Geometry: final body of the model. Coordinates: model frame, mm. Round coordinates to 2 decimals unless told otherwise and drop trailing zeros. Loops run counter-clockwise (first coordinate to the right, second up) from the corner with the lowest first, then second, coordinate; pieces in that order, holes last. Notation, with made-up numbers: M -16,33 L 16,33 A21 ccw 16,48 Z; hole C -20,76.25 d7. An arc over 180 degrees is marked long. Return JSON: item names as keys, results as strings.
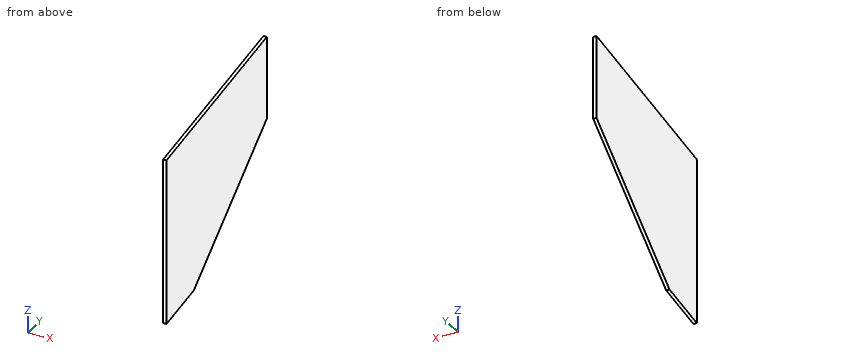
from build123d import *

# Parameters (mm, degrees)
BOSS_EXTRUDE1_DEPTH      = 1.27
BOSS_EXTRUDE1_DEPTH_BACK = 1.27


with BuildPart() as part:
    # Sketch1 → Boss-Extrude1 (new body, two sides)
    with BuildSketch(Plane(origin=(0, 0, 0), x_dir=(0, 0, -1), z_dir=(1, 0, 0))) as boss_extrude1_sk:
        Polygon((0, 0), (127, 0), (120.281942035, 38.1), (38.867120795, 139.7), (-24.632879205, 139.7), align=None)
    extrude(amount=BOSS_EXTRUDE1_DEPTH)
    extrude(boss_extrude1_sk.sketch, amount=-BOSS_EXTRUDE1_DEPTH_BACK)


solid = part.part
Q1. Section query A-A (x = -0.2). Output: boundary loops of the cut face in (y, z).
Determined:
{"outline": "M 0,-127 L 38.1,-120.28 L 139.7,-38.87 L 139.7,24.63 L 0,0 Z"}
Q2. Section query B-B (y = 46.5). Output: boundary loops of the cut face in (x, z), plus the area to 3 significant figures.
Determined:
{"outline": "M -1.27,-113.55 L 1.27,-113.55 L 1.27,8.2 L -1.27,8.2 Z", "area": "309 mm^2"}
Q3. Pin query (flat end, axial travel): pin 1 (1.5 mm diameter, centred on x = 0, y = 84, fed in from -Z). Return the tip coordinate at first contact, or that it passes through.
Determined:
{"pin 1": "stops at z = -84.1"}
Q4. Material intervals for L1, parallel to Z at x = -0.7, y = 120; L2, parallel to Y at x = -1, z = -78; L3, parallel to Z at x = 0.85, y = 27, sorted ascending.
Determined:
{"L1": "z = -54.65 to 21.16", "L2": "y = 0 to 90.86", "L3": "z = -122.24 to 4.76"}
Q5. Section query C-C (z = -60). Output: boundary loops of the cut face in (x, y).
Determined:
{"outline": "M -1.27,0 L 1.27,0 L 1.27,113.33 L -1.27,113.33 Z"}
